Geometry check sheet. Reference: the model listing, model coordinates, mm. A direction names the side the tool comes from. Give positions to 0.01 mm unless a question says otherwise; leave off trailing zeros. Order: outer loops, then holes, each group sorted by start corner. A loop starts at its lowest first (then second) coordinate and runs counter-clockwise, first axis right, second up. Notation, with made-up numbers: M 69.5,48 L 103.5,48 A24 cw 103.5,81 Z; hole C -37,-36.5 d11. An arc over 180 degrees is marked long. Answer as CSV lines item,"result". Start each with the question number.
Q1. Section check B-B, the plane x = 25.4. Record the boundary of the cut face in (y, z) (3 decimals).
Q2. Set-up check for faces 5 (the flat face through (6, -12.7, 26)), 6 (the flat face through (38.1, -38, 26)), 7 (the flat face through (19, 0, 43)): record each of +Z, -Z, +X, -X, +Y, -Y from which the full face is reachable in a straight line by a thin tool's end or side.
Q3. Section check C-C, the plane y = -31. Record the boundary of the cut face in (x, z), then the cut area to 3 significant figures.
Q4. Mould release check, pull along Z, two halves, no side actions. Record for faces 1 (the flat face through (25, -19, 0)), 2 (the cylindrical face through (25.58, -46.4, 16.95)), 3 (the flat face through (44, -12.7, 26)), 4 (the flat face through (25, -19, 50.8)): +Z half, -Z half, draft (parallel to the pull), parting line (faces both ways), or undercut.
Q5. Thickness scan on line 1 (Z direction, x = 29, y = -50); line 2 (Y direction, x = 41.5, z = 39); line 3 (X direction, y = -21.5, z = 32). Record the ranges inside material, lowest first.
Q6. Section check A-A, the plane z = 25.4. Record the boundary of the cut face in (x, y) (3 decimals).
Q7. Go/stop test with flat-tipped pins: pin 1 (15 mm diameter, centred on y = -52.5, z = 35.5, fed in from +X); pin 2 (12 mm diameter, centred on x = 33.5, z = 18, fed in from -Y); pin 3 (3 mm diameter, centred on x = 5.5, z = 6, fed in from -Y); pin 4 (10 mm diameter, centred on y = -52.5, z = 27, fed in from +X). Record where each tip stops, or that it passes through.
```python
from build123d import *

# Parameters (mm, degrees)
F0_W     = 50.8
F0_H     = 50.8
F1_DEPTH = 12.7
F2_W     = 12.7
F2_H     = 50.8
F3_DEPTH = 38.1
F5_DEPTH = 25.4
F6_R     = 9.525
F7_DEPTH = 25.4
F8_R     = 12.7
F9_DEPTH = 76.2
F10_R    = 2.54
F11_R    = 5.08


with BuildPart() as f1:
    # F0 (on Front) → F1 (new body)
    with BuildSketch(Plane.XZ):
        with Locations((25.4, 25.4)):
            Rectangle(F0_W, F0_H)
    extrude(amount=F1_DEPTH)

    # F2 (on face) → F3 (join)
    with BuildSketch(Plane.XZ.offset(12.7)):
        with Locations((19.05, 25.4)):
            Rectangle(F2_W, F2_H)
        with Locations((31.75, 25.4)):
            Rectangle(F2_W, F2_H)
    extrude(amount=F3_DEPTH)

    # F4 (on face) → F5 (join)
    with BuildSketch(Plane.YZ.offset(38.1)):
        with BuildLine():
            Line((-50.8, 0), (-50.8, 50.8))
            ThreePointArc((-50.8, 50.8), (-76.2, 25.4), (-50.8, 0))
        make_face()
    extrude(amount=-F5_DEPTH)

    # F6 (on face) → F7 (cut)
    with BuildSketch(Plane.YZ.offset(38.1)):
        with Locations((-50.8, 25.4)):
            Circle(F6_R)
    extrude(amount=-F7_DEPTH, mode=Mode.SUBTRACT)

    # F8 (on face) → F9 (join)
    with BuildSketch(Plane(origin=(0, 0, 0), x_dir=(-1, 0, 0), z_dir=(0, 1, 0))):
        with Locations((-25.4, 25.4)):
            Circle(F8_R)
    extrude(amount=F9_DEPTH)

    # F10
    f10_edges = [f1.edges().sort_by_distance(p)[0] for p in [
        (38.1, 76.2, 25.4),
    ]]
    fillet(f10_edges, radius=F10_R)

    # F11
    f11_edges = [f1.edges().sort_by_distance(p)[0] for p in [
        (12.7, 36.83, 25.4),
        (38.1, 73.66, 25.4),
        (38.1, 0, 25.4),
    ]]
    fillet(f11_edges, radius=F11_R)


solid = f1.part
```
Answer block:
1,outline,"M -50.8,0 L 0,0 L 0,7.62 A5.08 cw 5.08,12.7 L 73.66,12.7 A2.54 ccw 76.2,15.24 L 76.2,35.56 A2.54 ccw 73.66,38.1 L 5.08,38.1 A5.08 cw 0,43.18 L 0,50.8 L -50.8,50.8 A25.4 ccw Z; hole C -50.8,25.4 d19.05"
2,face 5,"+Z, -Z, -X, -Y"
2,face 6,"+Z, -Z, +X, -Y"
2,face 7,"+Y"
3,outline,"M 12.7,0 L 38.1,0 L 38.1,50.8 L 12.7,50.8 Z"
3,area,"1,290 mm2"
4,face 1,"-Z half"
4,face 2,"undercut"
4,face 3,"draft"
4,face 4,"+Z half"
5,line 1,"z = 0 to 15.91, 34.89 to 50.8"
5,line 2,"y = -12.7 to 0"
5,line 3,"x = 12.7 to 38.1"
6,outline,"M 0,-12.7 L 12.7,-12.7 L 12.7,-41.275 L 38.1,-41.275 L 38.1,-12.7 L 50.8,-12.7 L 50.8,0 L 43.18,0 A5.08 cw 38.1,5.08 L 38.1,73.66 A2.54 ccw 35.56,76.2 L 15.24,76.2 A2.54 ccw 12.7,73.66 L 12.7,5.08 A5.08 cw 7.62,0 L 0,0 Z; M 12.7,-76.2 L 38.1,-76.2 L 38.1,-60.325 L 12.7,-60.325 Z"
7,pin 1,"stops at x = 38.1"
7,pin 2,"stops at y = -76.16"
7,pin 3,"stops at y = -12.7"
7,pin 4,"passes through"
